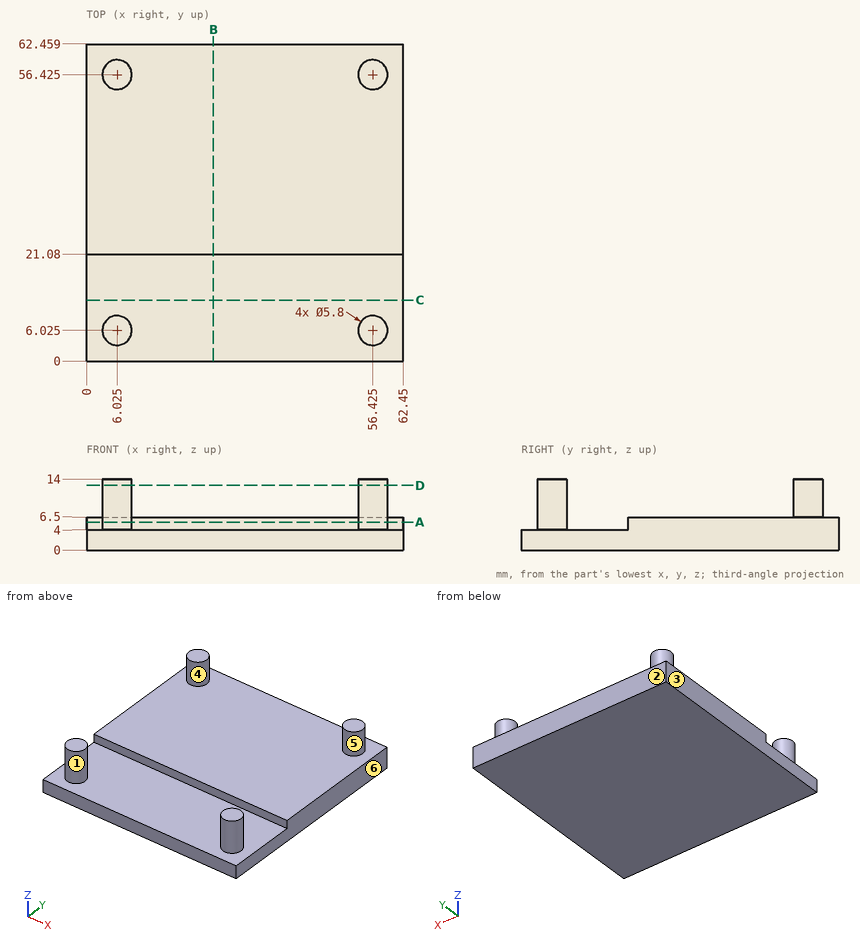
Print and shaded views of the part. All mm, measured from the part's lowest x, y and z. A direction names the side the tool comes from. Give positions to 0.01 mm unless a question says otherwise; leave off trailing zeros. Write each loop counter-clockwise with the first axis right and the second up, starting at its lowest first coordinate (ties: lowest second). Pieces come first, ordered by that corner, then holes. Notation, with made-up numbers: (-35, -34) - (3, -34) arc R13 ccw to (3, -20) - close; hole circle Ø2 at (-12.5, 86). An arc over 180 degrees is marked (long way). Put each result on its own line as item: value.
(1) Pull direction X, two halves, no side cores. Call the marked faces 1, 2, 3 and 4: released by +X, released by -X, zero draft, split by the parting line, or undercut.
Working result:
face 1: undercut
face 2: zero draft
face 3: released by -X
face 4: undercut
(2) Drop flat-ended pins along their axis: pin 1 Ø8 at (x, y) = (11, 19) entering from +Z; pin 2 Ø6 at (y, z) = (36, 11) entering from -X; pin 3 Ø6.5 at (x, y) = (35.5, 8.5) entering from +Z; pin 4 Ø4 at (y, z) = (10.5, 6.5) entering from -X (1 decimal). Give the stop position or say it passes through.
Working result:
pin 1: z = 6.5
pin 2: through
pin 3: z = 4
pin 4: x = 4.5
(3) Wall check: L1, parallel to Z at x = 31.5, y = 7; L2, parallel to X at y = 58.5, z = 7; L3, parallel to Z at x = 3.5, y = 36. Give the ranges that are in metal, low to high.
Working result:
L1: 0 to 4
L2: 4 to 8.05, 54.4 to 58.45
L3: 0 to 6.5
(4) Saw through at B-B (x = 25). List the corners of the cut face in (y, z), then the cut area to 3 significant figures.
Working result:
outline: (0, 0) - (62.46, 0) - (62.46, 6.5) - (21.08, 6.5) - (21.08, 4) - (0, 4) - close
area: 353 mm^2
(5) Saw through at A-A (z = 5.5). Count the separate pieces of the cut face and the enclosed holes in it, then the cut area to 3 significant figures.
Working result:
separate pieces: 3
enclosed holes: 0
area: 2,640 mm^2
(6) Tool access for the marked faces 5 and 6: list every direction of +Z, -Z, +X, -X, +Y, -Y with a clear straight run to the whole face (end or side of a thin tool).
Working result:
face 5: +Z
face 6: +Z, -Z, +X, +Y, -Y
(7) Saw through at C-C (y = 12). List the corners of the cut face in (x, z).
Working result:
outline: (0, 0) - (62.45, 0) - (62.45, 4) - (0, 4) - close
(8) Saw through at D-D (z = 12.75). List the corners of the cut face in (x, y) (1 decimal).
Working result:
outline: circle Ø5.8 at (6, 6); circle Ø5.8 at (6, 56.4); circle Ø5.8 at (56.4, 6); circle Ø5.8 at (56.4, 56.4)
